Check sheet for the modelled part. Datum: model origin and axes. Units: mm. Coordinates: 2 decimals unless noted, no trailing zeros. Loops run counter-clockwise (first coordinate to the right, second up) from the corner with the lowest first, then second, coordinate; pieces in that order, holes last. Notation, with made-up numbers: M 38.25,62.5 L 45.25,62.5 A19 ccw 45.25,89.5 Z; hole C 16,74.25 d2. An arc over 180 degrees is marked long. Return JSON: item names as keys, results as strings.
from build123d import *

# Parameters (mm, degrees)
SKETCH1_R           = 2
BOSS_EXTRUDE1_DEPTH = 4
SKETCH2_R           = 2.6
BOSS_EXTRUDE2_DEPTH = 1.75
CHAMFER1_SIZE       = 1


with BuildPart() as part:
    # Sketch1 → Boss-Extrude1 (new body)
    with BuildSketch(Plane.XY):
        Circle(SKETCH1_R)
    extrude(amount=BOSS_EXTRUDE1_DEPTH)

    # Sketch2 → Boss-Extrude2 (add)
    with BuildSketch(Plane(origin=(0, 0, 0), x_dir=(-1, 0, 0), z_dir=(0, 0, -1))):
        Circle(SKETCH2_R)
    extrude(amount=-BOSS_EXTRUDE2_DEPTH)

    # Chamfer1
    # the kernel refuses this chamfer: 1 mm, written as the material it takes off along each edge
    with BuildSketch(Plane(origin=(0, 0, 1.75), x_dir=(-1, 0, 0), z_dir=(0, -1, 0))) as chamfer1_piece_1_section:
        Polygon((2.6, CHAMFER1_SIZE), (2.6 - CHAMFER1_SIZE, 0), (2.6, 0), align=None)
    chamfer1_piece_1 = revolve(axis=Axis((0, 0, 1.75), (0, 0, -1)), mode=Mode.PRIVATE)
    chamfer1_piece_1 = chamfer1_piece_1 - Plane(origin=(0, 0, 1.049223844), x_dir=(1, 0, 0), z_dir=(0, 0, -1)) * Cylinder(2, 11, mode=Mode.PRIVATE)
    add(chamfer1_piece_1, mode=Mode.SUBTRACT)


solid = part.part
1) Section check C-C on z = 3.6. Record the cut outline in (x, y).
Answers:
{"outline": "C 0,0 d4"}
2) Section check A-A on y = 0. Record the cut outline in (x, z).
Answers:
{"outline": "M -2.6,0 L 2.6,0 L 2.6,0.75 L 2,1.35 L 2,4 L -2,4 L -2,1.35 L -2.6,0.75 Z"}
3) Scan lines: line 1 along Y through (x, z) = (0, 1.65); line 2 along Y through (x, z) = (2.2, 0.5); line 3 along X through (y, z) = (0.35, 0.6). Record each from-to range of solid material in increasing order. Write a range as [from, to].
Answers:
{"line 1": "[-2, 2]", "line 2": "[-1.39, 1.39]", "line 3": "[-2.58, 2.58]"}
